Part print with two shaded views. Sizes in mm from the minimum x, y, z corner. A direction names the side the tool comes from. Give positions to 0.01 mm unless a question says otherwise; leave off trailing zeros. Order: outer loops, then holes, each group sorted by start corner. A loop starts at its lowest first (then second) coordinate and runs counter-clockwise, first axis right, second up. Notation, with made-up numbers: M 46,55.25 L 54,55.25 A22 ccw 54,90.25 Z; hole C 55.5,-9.5 d11. An arc over 180 degrees is marked long. Write each question's results on one line, items separated by ' | '. Start each with the question number.
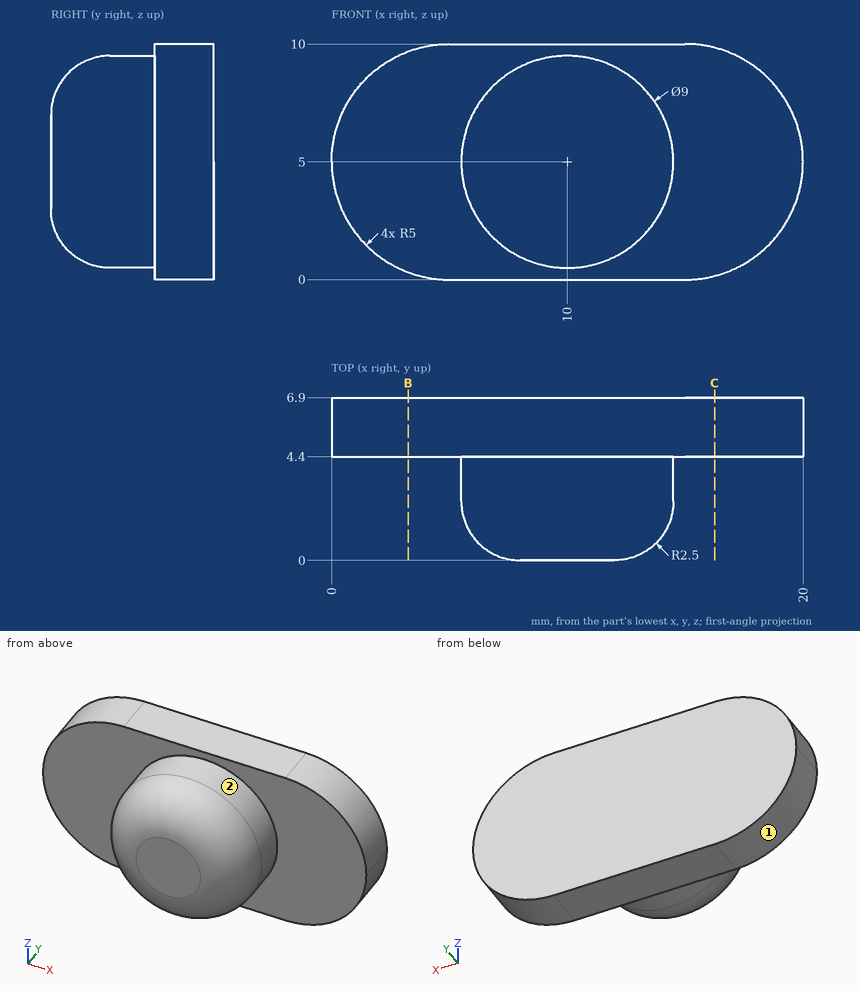
(1) Probe L1, parallel to Y at x = 18, z = 7.25; L2, parallel to X at y = 5.25, z = 7; L3, parallel to Y at x = 13.5, z = 3.25. List the from-to ranges inside material, lowest first.
(2) Drop flat-ended pins along their axis: P1, Ø1, axis at y = 3.5, z = 1.5, coming from the +X side; P2, Ø4, axis at x = 2.5, y = 1.5, coming from the +Z side; P3, Ø2, axis at x = 17, z = 8, coming from the -Y side. Give the stop position or say it passes through.
(3) Saw through at C-C on x = 16.25. Give the cut face in (y, z).
(4) Saw through at B-B on x = 3.25. Give the cut face in (y, z), plus the area to 3 significant figures.
(5) Tool access for the marked faces 1 and 2: list every direction of +Z, -Z, +X, -X, +Y, -Y with a clear straight run to the whole face (end or side of a thin tool).
Taken from the geometry:
1) L1: y = 4.4 to 6.9 | L2: x = 0.42 to 19.58 | L3: y = 0.89 to 6.9
2) P1: stops at x = 13.35 | P2: passes through | P3: stops at y = 4.4
3) outline: M 4.4,0.16 L 6.9,0.16 L 6.9,9.84 L 4.4,9.84 Z
4) outline: M 4.4,0.32 L 6.9,0.32 L 6.9,9.68 L 4.4,9.68 Z | area: 23.4 mm²
5) face 1: -Z, -X, +Y, -Y | face 2: -Y
